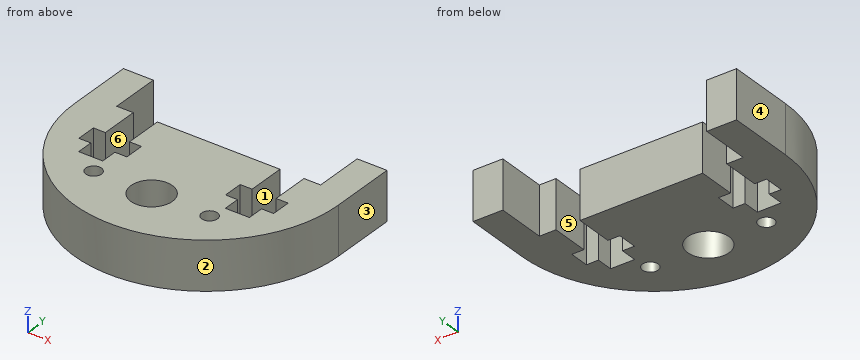
```python
from build123d import *

# Parameters (mm, degrees)
MODEL_R             = 0.95
MODEL_R_2           = 2.49989274
BOSS_EXTRUDE2_DEPTH = 5.85


with BuildPart() as part:
    # Model → Boss-Extrude2 (new body)
    with BuildSketch(Plane.XY):
        with BuildLine():
            Line((553.509477136, 558.532469), (546.109477136, 558.532469))
            Line((546.109477136, 558.532469), (546.109477136, 553.961751207))
            Line((546.109477136, 553.961751207), (547.559476844, 553.962671766))
            Line((547.559476844, 553.962671766), (547.559476844, 551.562620711))
            Line((547.559476844, 551.562620711), (546.109477111, 551.563500787))
            Line((546.109477111, 551.563500787), (546.109477111, 549.563500787))
            Line((546.109477111, 549.563500787), (543.209383557, 549.573000091))
            Line((543.209383557, 549.573000091), (543.209383557, 551.573000091))
            Line((543.209383557, 551.573000091), (541.759477136, 551.556526783))
            Line((541.759477136, 551.556526783), (541.759477136, 553.956577839))
            Line((541.759477136, 553.956577839), (543.209477136, 553.956563))
            Line((543.209477136, 553.956563), (543.209477136, 558.532469))
            Line((543.209477136, 558.532469), (541.209477136, 558.532469))
            Line((541.209477136, 558.532469), (541.209477136, 564.532469))
            Line((541.209477136, 564.532469), (537.609477136, 564.532469))
            Line((537.609477136, 564.532469), (537.609477136, 556.532469))
            ThreePointArc((537.609477136, 556.532469), (553.509477136, 540.632469), (569.409477136, 556.532469))
            Line((569.409477136, 556.532469), (569.409477136, 564.532469))
            Line((569.409477136, 564.532469), (565.809477136, 564.532469))
            Line((565.809477136, 564.532469), (565.809477136, 558.532469))
            Line((565.809477136, 558.532469), (563.809477136, 558.532469))
            Line((563.809477136, 558.532469), (563.809477136, 553.956563))
            Line((563.809477136, 553.956563), (565.259477136, 553.956577839))
            Line((565.259477136, 553.956577839), (565.259477136, 551.556526783))
            Line((565.259477136, 551.556526783), (563.809570715, 551.573000091))
            Line((563.809570715, 551.573000091), (563.809570715, 549.573000091))
            Line((563.809570715, 549.573000091), (560.909477161, 549.563500787))
            Line((560.909477161, 549.563500787), (560.909477161, 551.563500787))
            Line((560.909477161, 551.563500787), (559.459477428, 551.562620711))
            Line((559.459477428, 551.562620711), (559.459477428, 553.962671766))
            Line((559.459477428, 553.962671766), (560.909477136, 553.961751207))
            Line((560.909477136, 553.961751207), (560.909477136, 558.532469))
            Line((560.909477136, 558.532469), (553.509477136, 558.532469))
        make_face()
        with Locations((546.509477136, 547.532469)):
            Circle(MODEL_R, mode=Mode.SUBTRACT)
        with Locations((553.509477136, 547.532469)):
            Circle(MODEL_R_2, mode=Mode.SUBTRACT)
        with Locations((560.509477136, 547.532469)):
            Circle(MODEL_R, mode=Mode.SUBTRACT)
    extrude(amount=BOSS_EXTRUDE2_DEPTH)


solid = part.part
```
Here's how the part is built. I have some questions about the finished solid (model axes, mm). Face numbers are marked on the shaded views. A direction names the side the tool comes from. Give positions to 0.01 mm unless a question says otherwise; leave off trailing zeros. Loops run counter-clockwise (first coordinate to the right, second up) from the corner with the lowest first, then second, coordinate; pieces in that order, holes last. Notation, with made-up numbers: M 21.25,53.25 L 60.25,53.25 A28 cw 60.25,74.25 Z; hole C 11,-26 d8. An arc over 180 degrees is marked long. Put each result on its own line as item: value. Start each with the question number.
(1) I need wall thicknesses on line 1 along X through (y, z) = (557, 2.45); line 2 along X through (y, z) = (547, 5.55); line 3 along X through (y, z) = (559.5, 2.35). Which ranges of each line are inside material? Lowest first, please. Write a range as [from, to].
(2) I want a section at A-A on y = 559.5. Please give me the cut outline in (x, z).
(3) I want a section at C-C on z = 2.15. State how many separate pieces and enclosed holes the cut face has, then the cut area to 3 significant figures.
(4) For the marked faces 1 and 2, which set-ups out of +Z, -Z, +X, -X, +Y, -Y let a thin tool reach every point of the face, with its end or its side?
(5) I want a section at D-D on x = 550. Please give me the cut outline in (y, z).
(6) Will these pins go through, and if not, where does the flat tip stop? pin 1 Ø4 at (x, y) = (553.51, 547.53) entering from -Z; pin 2 Ø0.7 at (x, z) = (542, 4) entering from -Y; pin 3 Ø0.6 at (y, z) = (550, 3.5) entering from -X; pin 4 Ø1.2 at (y, z) = (552.5, 3.5) entering from +X.
(7) I want a section at B-B on y = 553. Please give me the cut outline in (x, z), then the cut area to 3 significant figures.
(8) If we mould it in two halves opening along X, with no side actions, what happens to the marked faces 3, 4, 5 and 6? For each: +X half, -X half, draft (parallel to the pull), parting line (faces both ways), or undercut.
Answer block:
1. line 1: [537.61, 543.21], [546.11, 560.91], [563.81, 569.41]
1. line 2: [540.78, 545.72], [547.3, 551.07], [555.95, 559.72], [561.3, 566.24]
1. line 3: [537.61, 541.21], [565.81, 569.41]
2. outline: M 537.61,0 L 541.21,0 L 541.21,5.85 L 537.61,5.85 Z; M 565.81,0 L 569.41,0 L 569.41,5.85 L 565.81,5.85 Z
3. separate pieces: 1
3. enclosed holes: 3
3. area: 413 mm^2
4. face 1: +Z, -Z, +Y
4. face 2: +Z, -Z, -Y
5. outline: M 541.02,0 L 558.53,0 L 558.53,5.85 L 541.02,5.85 Z
6. pin 1: through
6. pin 2: y = 545.21
6. pin 3: x = 538.88
6. pin 4: x = 569.03
7. outline: M 538.01,0 L 541.76,0 L 541.76,5.85 L 538.01,5.85 Z; M 547.56,0 L 559.46,0 L 559.46,5.85 L 547.56,5.85 Z; M 565.26,0 L 569.01,0 L 569.01,5.85 L 565.26,5.85 Z
7. area: 114 mm^2
8. face 3: +X half
8. face 4: -X half
8. face 5: undercut
8. face 6: undercut
